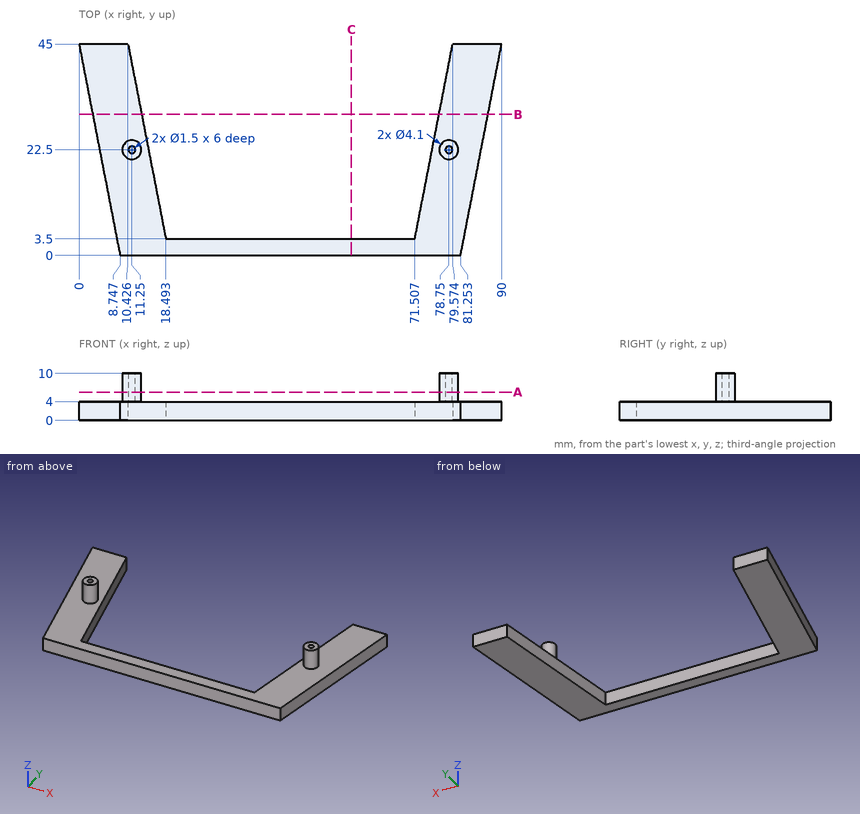
Here's the drawing with two shaded views (mm, measured from the low corner). I have some questions. Coordinates: 2 decimals unless noted, no trailing zeros. Order: outer loops, then holes, each group sorted by start corner. A loop starts at its lowest first (then second) coordinate and runs counter-clockwise, first axis right, second up.
Item 1: I need wall thicknesses on line 1 (Y direction, x = 11.25, z = 8.75); line 2 (X direction, y = 34, z = 1) (1 decimal); line 3 (Z direction, x = 11, y = 31). Which ranges of each line are inside material? Lowest first, please.
Result sheet:
line 1: y = 20.45 to 21.75, 23.25 to 24.55
line 2: x = 2.1 to 12.6, 77.4 to 87.9
line 3: z = 0 to 4
Item 2: For P1, Ø6, axis at y = 7.5, z = 6, coming from the +X side (1 decimal); P2, Ø1.2, axis at x = 38.5, z = 2.5, coming from the +Y side; P3, Ø4, axis at y = 35, z = 4, coming from the -X side (1 decimal); P4, Ø0.8, axis at x = 79, y = 22, coming from the +Z side, each with a flat end and sliding along its axis, tell me the tip position at first contact or that it passes through.
Result sheet:
P1: stops at x = 83.1
P2: stops at y = 3.5
P3: stops at x = 1.6
P4: stops at z = 10
Item 3: If we section it at B-B on y = 30: List the corners of the cut face in (x, z) for me (1 decimal).
Result sheet:
outline: (2.9, 0) - (13.3, 0) - (13.3, 4) - (2.9, 4) - close; (76.7, 0) - (87.1, 0) - (87.1, 4) - (76.7, 4) - close
Item 4: If we section it at C-C on x = 58: List the corners of the cut face in (y, z) for me, plus the area to 3 significant figures.
Result sheet:
outline: (0, 0) - (3.5, 0) - (3.5, 4) - (0, 4) - close
area: 14.0 mm2
Item 5: If we section it at A-A on z = 6: List the corners of the cut face in (x, y) for me.
Result sheet:
outline: circle Ø4.1 at (11.25, 22.5); circle Ø4.1 at (78.75, 22.5); hole circle Ø1.5 at (11.25, 22.5); hole circle Ø1.5 at (78.75, 22.5)
